Geometry check sheet. Reference: drawing and pictorial views, mm from the part's lowest x, y, z. A direction names the side the tool comes from. Round coordinates to 2 decimals unless told otherwise and drop trailing zeros. Write each loop counter-clockwise with the first axis right and the second up, starting at its lowest first coordinate (ties: lowest second). Pieces come first, ordered by that corner, then holes. Notation, with made-up numbers: (46.5, 32.25) - (68.5, 32.25) arc R22 cw to (68.5, 49.25) - close; hole circle Ø4 at (-20.5, -8.5). An arc over 180 degrees is marked (long way). Use one line per item in the form item = value. Start each with the question number.
1) Set-up check for the marked faces 1, 2 and 3: record each of +Z, -Z, +X, -X, +Y, -Y from which the full face is reachable in a straight line by a thin tool's end or side.
2) Scan lines: probe 1 along Z at (x, y) = (12.5, 8.25); probe 2 along Z at (x, y) = (6, 11.25); probe 3 along X at (y, z) = (6.75, 8.75). Record each from-to range of solid material in increasing order.
3) Section check A-A (y = 7). Record the boundary of the cut face in (x, z), then the cut area to 3 significant figures.
4) Gauge pin test, flat ends, axial feed: P1, Ø6, axis at x = 3.5, y = 10, coming from the -Z side; P2, Ø2, axis at y = 2.5, z = 6.5, coming from the -X side; P3, Ø4, axis at y = 7, z = 2, coming from the +X side; P4, Ø4, axis at x = 4.5, z = 6.5, coming from the -Y side. Record the tip position at first contact, or that the pin passes through.
5) Section check D-D (y = 2.25). Record the boundary of the cut face in (x, z).
6) Section check C-C (z = 11.5). Record the boundary of the cut face in (x, y), then the cut area to 3 significant figures.
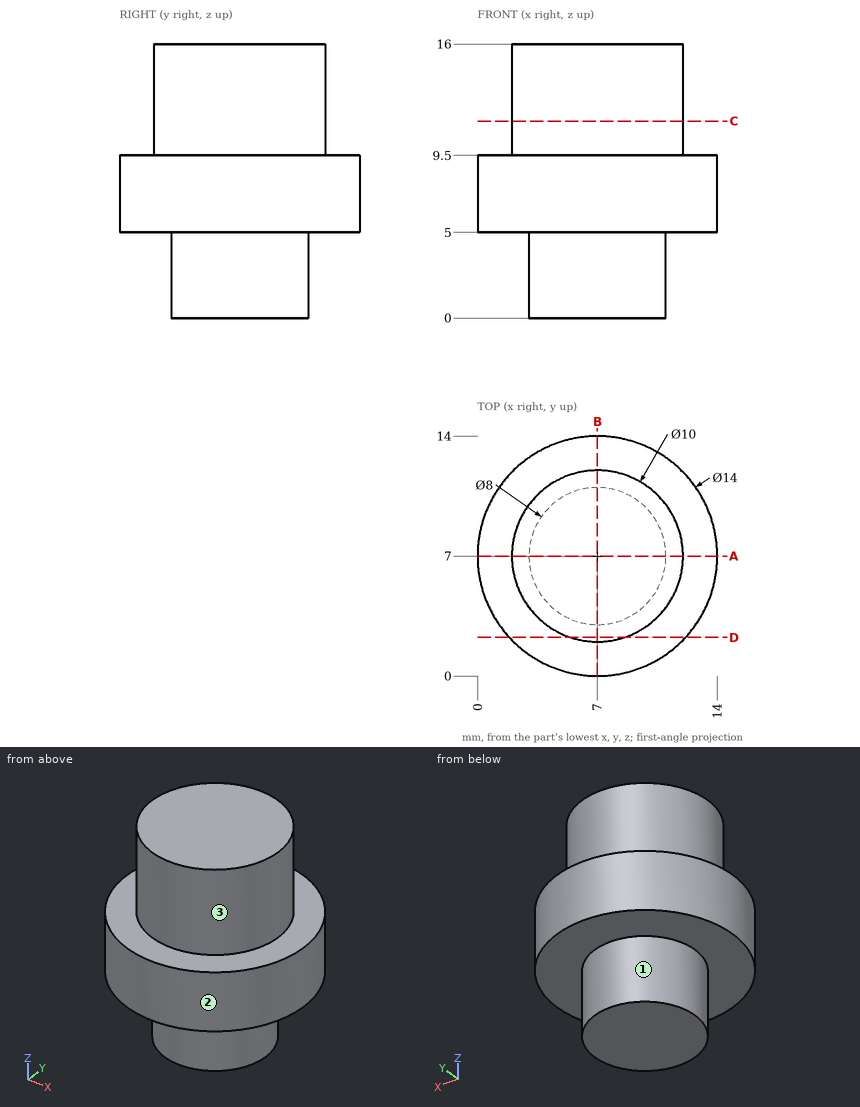
Results are:
q1.face_1 = -Z
q1.face_2 = +Z, -Z
q1.face_3 = +Z
q2.probe_1 = 5 to 9.5
q2.probe_2 = 5 to 16
q2.probe_3 = 0 to 14
q3.outline = (0, 5) - (3, 5) - (3, 0) - (11, 0) - (11, 5) - (14, 5) - (14, 9.5) - (12, 9.5) - (12, 16) - (2, 16) - (2, 9.5) - (0, 9.5) - close
q3.area = 168 mm²
q4.P1 = 0
q4.P2 = 0.94
q4.P3 = 11
q4.P4 = 0.02
q5.outline = (1.86, 5) - (12.14, 5) - (12.14, 9.5) - (8.56, 9.5) - (8.56, 16) - (5.44, 16) - (5.44, 9.5) - (1.86, 9.5) - close
q6.outline = circle Ø10 at (7, 7)
q6.area = 78.5 mm²
